Geometry check sheet. Reference: the model listing, model coordinates, mm. Face numbers are marked on the shaded views. A direction names the side the tool comes from. Coordinates: 2 decimals unless noted, no trailing zeros. Loops run counter-clockwise (first coordinate to the right, second up) from the corner with the lowest first, then second, coordinate; pieces in that order, holes last. Notation, with made-up numbers: (59, -36) -> (91, -36) arc R3 cw to (91, -31) -> close; hole circle Ø8 at (-32.75, -19). An arc over 180 degrees is marked (long way). Answer as a JSON object with one key per item and string values.
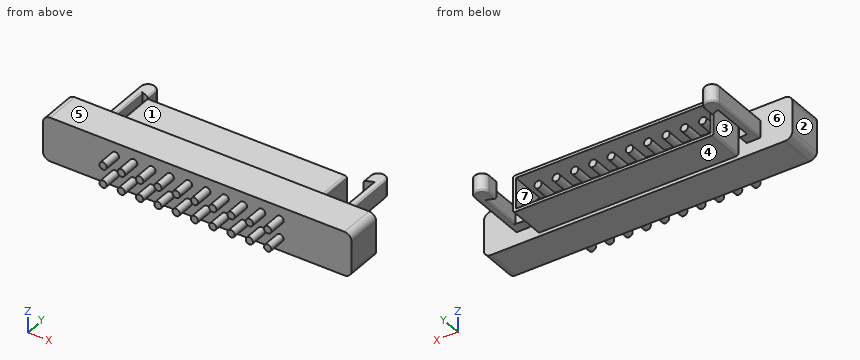
from build123d import *

# Parameters (mm, degrees)
SKETCH_2_W             = 38.1
SKETCH_2_H             = 1
EXTRUDE_1_DEPTH        = 5.08
SKETCH_3_R             = 0.514113779
SKETCH_3_R_2           = 0.502427848
EXTRUDE_2_DEPTH        = 2.5
PATTERN_LINEAR_1_COUNT = 10
PATTERN_LINEAR_1_PITCH = 2.54
SKETCH_4_W             = 44.198683318
SKETCH_4_H             = 8.471214157
CUT_EXTRUDE_1_DEPTH    = 5.08
EXTRUDE_START          = 6
SKETCH_5_R             = 0.502427848
SKETCH_5_R_2           = 0.514113779
EXTRUDE_3_DEPTH        = 6
SKETCH_6_W             = 51.24
SKETCH_6_H             = 6.08
EXTRUDE_4_DEPTH        = 2.4
SKETCH_7_W             = 27.84
SKETCH_7_H             = 5.08
SKETCH_7_W_2           = 27.04
SKETCH_7_H_2           = 4.28
EXTRUDE_6_DEPTH        = 7.5
SKETCH_8_W             = 51.24
SKETCH_8_H             = 6.08
EXTRUDE_7_DEPTH        = 2.6
EXTRUDE_8_DEPTH        = 1.25
EXTRUDE_8_DEPTH_BACK   = 1.25
FILLET_1_R             = 0.3
FILLET_2_R             = 0.2
SKETCH_10_W            = 6.08
SKETCH_10_H            = 5
CUT_EXTRUDE_2_DEPTH    = 13.4
SKETCH_11_W            = 6.08
SKETCH_11_H            = 5
EXTRUDE_9_DEPTH        = 2.5
SKETCH_12_W            = 6.08
SKETCH_12_H            = 5
EXTRUDE_10_DEPTH       = 2.5
FILLET_3_R             = 1


with BuildPart() as part:
    # Эскиз2 → Вытянуть1 (new body)
    with BuildSketch(Plane.XY):
        Polygon((0, 0), (41.24, 0), (41.24, 2.54), (40.94, 2.54), (40.94, 3.34), (41.24, 3.34), (41.24, 7.62), (0, 7.62), (0, 3.34), (0.3, 3.34), (0.3, 2.54), (0, 2.54), align=None)
        with Locations((20.62, 5.5)):
            Rectangle(SKETCH_2_W, SKETCH_2_H, mode=Mode.SUBTRACT)
    extrude(amount=EXTRUDE_1_DEPTH)

    # Эскиз3 → Вытянуть2 (add)
    with BuildSketch(Plane.XZ):
        with Locations(Location((2.54, 3.81, 0), (0, 0, 90))):
            Circle(SKETCH_3_R)
        with Locations(Location((2.54, 1.27, 0), (0, 0, 90))):
            Circle(SKETCH_3_R_2)
    extrude_2 = extrude(amount=EXTRUDE_2_DEPTH)

    # Линейный массив1: Вытянуть2 ×10
    with Locations(*[(i * PATTERN_LINEAR_1_PITCH, 0, 0) for i in range(1, PATTERN_LINEAR_1_COUNT)]):
        add(extrude_2)

    # Эскиз4 → Вырез-Вытянуть1 (cut)
    with BuildSketch(Plane(origin=(0, 7.62, 0), x_dir=(-1, 0, 0), z_dir=(0, 1, 0))):
        with Locations((-20.961321946, 2.444099463)):
            Rectangle(SKETCH_4_W, SKETCH_4_H)
    extrude(amount=-CUT_EXTRUDE_1_DEPTH, mode=Mode.SUBTRACT)

    # Эскиз5 → Вытянуть3 (add)
    with BuildSketch(Plane(origin=(0, 2.54, 0), x_dir=(-1, 0, 0), z_dir=(0, 1, 0)).offset(EXTRUDE_START)):
        with Locations(Location((-15.24, 1.27, 0), (0, 0, 90))):
            Circle(SKETCH_5_R)
        with Locations(Location((-15.24, 3.81, 0), (0, 0, 90))):
            Circle(SKETCH_5_R_2)
        with Locations(Location((-17.78, 1.27, 0), (0, 0, 90))):
            Circle(SKETCH_5_R)
        with Locations(Location((-17.78, 3.81, 0), (0, 0, 90))):
            Circle(SKETCH_5_R_2)
        with Locations(Location((-20.32, 1.27, 0), (0, 0, 90))):
            Circle(SKETCH_5_R)
        with Locations(Location((-20.32, 3.81, 0), (0, 0, 90))):
            Circle(SKETCH_5_R_2)
        with Locations(Location((-22.86, 1.27, 0), (0, 0, 90))):
            Circle(SKETCH_5_R)
        with Locations(Location((-12.7, 3.81, 0), (0, 0, 90))):
            Circle(SKETCH_5_R_2)
        with Locations(Location((-10.16, 3.81, 0), (0, 0, 90))):
            Circle(SKETCH_5_R_2)
        with Locations(Location((-7.62, 3.81, 0), (0, 0, 90))):
            Circle(SKETCH_5_R_2)
        with Locations(Location((-5.08, 3.81, 0), (0, 0, 90))):
            Circle(SKETCH_5_R_2)
        with Locations(Location((-2.54, 3.81, 0), (0, 0, 90))):
            Circle(SKETCH_5_R_2)
        with Locations(Location((-2.54, 1.27, 0), (0, 0, 90))):
            Circle(SKETCH_5_R)
        with Locations(Location((-5.08, 1.27, 0), (0, 0, 90))):
            Circle(SKETCH_5_R)
        with Locations(Location((-7.62, 1.27, 0), (0, 0, 90))):
            Circle(SKETCH_5_R)
        with Locations(Location((-10.16, 1.27, 0), (0, 0, 90))):
            Circle(SKETCH_5_R)
        with Locations(Location((-12.7, 1.27, 0), (0, 0, 90))):
            Circle(SKETCH_5_R)
        with Locations(Location((-22.86, 3.81, 0), (0, 0, 90))):
            Circle(SKETCH_5_R_2)
        with Locations(Location((-25.4, 1.27, 0), (0, 0, 90))):
            Circle(SKETCH_5_R)
        with Locations(Location((-25.4, 3.81, 0), (0, 0, 90))):
            Circle(SKETCH_5_R_2)
    extrude(amount=-EXTRUDE_3_DEPTH)

    # Эскиз6 → Вытянуть4 (add)
    with BuildSketch(Plane.XZ):
        with Locations((20.62, 2.54)):
            Rectangle(SKETCH_6_W, SKETCH_6_H)
    extrude(amount=-EXTRUDE_4_DEPTH)

    # Эскиз7 → Вытянуть6 (add)
    with BuildSketch(Plane(origin=(0, 2.54, 0), x_dir=(-1, 0, 0), z_dir=(0, 1, 0))):
        with Locations((-13.92, 2.54)):
            Rectangle(SKETCH_7_W, SKETCH_7_H)
        with Locations((-13.92, 2.54)):
            Rectangle(SKETCH_7_W_2, SKETCH_7_H_2, mode=Mode.SUBTRACT)
    extrude(amount=EXTRUDE_6_DEPTH)

    # Эскиз8 → Вытянуть7 (add)
    with BuildSketch(Plane(origin=(0, 2.4, 0), x_dir=(-1, 0, 0), z_dir=(0, 1, 0))):
        with Locations((-20.62, 2.54)):
            Rectangle(SKETCH_8_W, SKETCH_8_H)
    extrude(amount=EXTRUDE_7_DEPTH)

    # Эскиз9 → Вытянуть8 (add, two sides: drawn at the far end of the back side and taken through both)
    with BuildSketch(Plane.XY.offset(2.54).offset(-EXTRUDE_8_DEPTH_BACK)):
        with BuildLine():
            Line((-3.08, 2.225086662), (-1.038499325, 2.225086662))
            Line((-1.038499325, 2.225086662), (-1.038499325, 6.369811339))
            Line((-1.038499325, 6.369811339), (-2.112614583, 6.464724855))
            Line((-2.112614583, 6.464724855), (-2.112614583, 12.347438775))
            Line((-2.112614583, 12.347438775), (-1.038499325, 11.921130469))
            Line((-1.038499325, 11.921130469), (-1.038499325, 13.347619973))
            ThreePointArc((-1.038499325, 13.347619973), (-2.059249663, 14.368370311), (-3.08, 13.347619973))
            Line((-3.08, 13.347619973), (-3.08, 2.225086662))
        make_face()
        with BuildLine():
            Line((28.878499325, 11.921130469), (28.878499325, 13.347619973))
            ThreePointArc((28.878499325, 13.347619973), (29.899249663, 14.368370311), (30.92, 13.347619973))
            Line((30.92, 13.347619973), (30.92, 2.225086662))
            Line((30.92, 2.225086662), (28.878499325, 2.225086662))
            Line((28.878499325, 2.225086662), (28.878499325, 6.369811339))
            Line((28.878499325, 6.369811339), (29.952614583, 6.464724855))
            Line((29.952614583, 6.464724855), (29.952614583, 12.347438775))
            Line((29.952614583, 12.347438775), (28.878499325, 11.921130469))
        make_face()
    extrude(amount=EXTRUDE_8_DEPTH + EXTRUDE_8_DEPTH_BACK)

    # Скругление1
    fillet_1_edges = [part.edges().sort_by_distance(p)[0] for p in [
        (0, 7.52, 0),
        (27.84, 7.52, 5.08),
        (27.84, 7.52, 0),
        (0, 7.52, 5.08),
    ]]
    fillet(fillet_1_edges, radius=FILLET_1_R)

    # Скругление2
    fillet_2_edges = [part.edges().sort_by_distance(p)[0] for p in [
        (-3.08, 9.173809987, 1.29),
        (-1.038499325, 5.684905669, 1.29),
        (-3.08, 9.173809987, 3.79),
        (-1.038499325, 5.684905669, 3.79),
        (-2.112614583, 9.406081815, 3.79),
        (-1.038499325, 12.634375221, 3.79),
        (-2.059249663, 14.368370311, 3.79),
        (-2.112614583, 9.406081815, 1.29),
        (-1.038499325, 12.634375221, 1.29),
        (-2.059249663, 14.368370311, 1.29),
        (28.878499325, 5.684905669, 1.29),
        (30.92, 9.173809987, 1.29),
        (30.92, 9.173809987, 3.79),
        (29.899249663, 14.368370311, 3.79),
        (28.878499325, 12.634375221, 3.79),
        (29.952614583, 9.406081815, 3.79),
        (28.878499325, 5.684905669, 3.79),
        (29.899249663, 14.368370311, 1.29),
        (28.878499325, 12.634375221, 1.29),
        (29.952614583, 9.406081815, 1.29),
    ]]
    fillet(fillet_2_edges, radius=FILLET_2_R)

    # Эскиз10 → Вырез-Вытянуть2 (cut)
    with BuildSketch(Plane(origin=(46.24, 0, 0), x_dir=(0, 0, -1), z_dir=(1, 0, 0))):
        with Locations((-2.54, 2.5)):
            Rectangle(SKETCH_10_W, SKETCH_10_H)
    extrude(amount=-CUT_EXTRUDE_2_DEPTH, mode=Mode.SUBTRACT)

    # Эскиз11 → Вытянуть9 (add)
    with BuildSketch(Plane(origin=(32.84, 0, 0), x_dir=(0, 0, -1), z_dir=(1, 0, 0))):
        with Locations((-2.54, 2.5)):
            Rectangle(SKETCH_11_W, SKETCH_11_H)
    extrude(amount=EXTRUDE_9_DEPTH)

    # Эскиз12 → Вытянуть10 (add)
    with BuildSketch(Plane.ZY.offset(5)):
        with Locations((2.54, 2.5)):
            Rectangle(SKETCH_12_W, SKETCH_12_H)
    extrude(amount=EXTRUDE_10_DEPTH)

    # Скругление3
    fillet_3_edges = [part.edges().sort_by_distance(p)[0] for p in [
        (35.34, 2.5, 5.58),
        (35.34, 2.5, -0.5),
        (-7.5, 2.5, -0.5),
        (-7.5, 2.5, 5.58),
    ]]
    fillet(fillet_3_edges, radius=FILLET_3_R)


solid = part.part
1. Section check B-B, the plane x = 7.62. Record the boundary of the cut face in (y, z), then the cut area to 3 significant figures.
Evaluation:
{"outline": "(-2.5, 0.77) -> (0, 0.77) -> (0, -0.5) -> (5, -0.5) -> (5, 0) -> (10.04, 0) -> (10.04, 0.4) -> (5, 0.4) -> (5, 0.77) -> (8.54, 0.77) -> (8.54, 1.77) -> (5, 1.77) -> (5, 3.3) -> (8.54, 3.3) -> (8.54, 4.32) -> (5, 4.32) -> (5, 4.68) -> (10.04, 4.68) -> (10.04, 5.08) -> (5, 5.08) -> (5, 5.58) -> (0, 5.58) -> (0, 4.32) -> (-2.5, 4.32) -> (-2.5, 3.3) -> (0, 3.3) -> (0, 1.77) -> (-2.5, 1.77) -> close", "area": "46.7 mm^2"}
2. Depth check by flat-ended pin: P1, Ø1, axis at y = 9.5, z = 2.5, coming from the -X side; P2, Ø1, axis at x = 2, z = 2.5, coming from the +Y side; P3, Ø2.5, axis at x = 12.5, y = 8.5, coming from the -Z side. Enter the tip coordinate at first touch or a pass-through.
Evaluation:
{"P1": "stops at x = -3.08", "P2": "stops at y = 5", "P3": "stops at z = 0"}
3. Thickness scan on probe 1 along X at (y, z) = (9.5, 2.25); probe 2 along X at (y, z) = (10.5, 1.5); probe 3 along X at (y, z) = (10, 1). Record the ranges inside material, lowest first. Write a range as from..to.
Evaluation:
{"probe 1": "x = -3.08..-2.11, 0..0.4, 27.44..27.84, 29.95..30.92", "probe 2": "x = -3.08..-2.11, 29.95..30.92", "probe 3": "x = 0..0.4, 27.44..27.84"}
4. Tool access check on the marked faces 1, 2 and 3. Record the directions out of +Z, -Z, +X, -X, +Y, -Y that give a thin tool (end or side, any length) a straight path to the whole face; none if there is none.
Evaluation:
{"face 1": "+Z, +X, -X, +Y", "face 2": "+Z, -Z, -X, +Y, -Y", "face 3": "+Z, -Z, +Y"}
5. Section check C-C, the plane x = 14. Record the boundary of the cut face in (y, z).
Evaluation:
{"outline": "(0, -0.5) -> (5, -0.5) -> (5, 0) -> (10.04, 0) -> (10.04, 0.4) -> (5, 0.4) -> (5, 4.68) -> (10.04, 4.68) -> (10.04, 5.08) -> (5, 5.08) -> (5, 5.58) -> (0, 5.58) -> close"}
6. Section check A-A, the plane y = 11. Record the boundary of the cut face in (x, z), then the cut area to 3 significant figures.
Evaluation:
{"outline": "(-3.08, 1.49) arc R0.2 ccw to (-2.88, 1.29) -> (-2.31, 1.29) arc R0.2 ccw to (-2.11, 1.49) -> (-2.11, 3.59) arc R0.2 ccw to (-2.31, 3.79) -> (-2.88, 3.79) arc R0.2 ccw to (-3.08, 3.59) -> close; (29.95, 1.49) arc R0.2 ccw to (30.15, 1.29) -> (30.72, 1.29) arc R0.2 ccw to (30.92, 1.49) -> (30.92, 3.59) arc R0.2 ccw to (30.72, 3.79) -> (30.15, 3.79) arc R0.2 ccw to (29.95, 3.59) -> close", "area": "4.77 mm^2"}
7. Mould release check, pull along Z, two halves, no side actions. Record for the marked faces 4, 5, 6 and 7: released by +Z, released by -Z, zero draft, split by the parting line, or undercut.
Evaluation:
{"face 4": "released by -Z", "face 5": "released by +Z", "face 6": "zero draft", "face 7": "undercut"}
8. Section check D-D, the plane x = -0.5. Record the boundary of the cut face in (y, z).
Evaluation:
{"outline": "(0, -0.5) -> (5, -0.5) -> (5, 5.58) -> (0, 5.58) -> close"}
